Autodesk Inventor part; units mm, degrees
ref_plane "YZ Plane" through (0, 0, 0) normal (1, 0, 0) x (0, 1, 0)
ref_plane "XZ Plane" through (0, 0, 0) normal (0, 1, 0) x (-1, 0, 0)
ref_plane "XY Plane" through (0, 0, 0) normal (0, 0, 1) x (1, 0, 0)
sketch "Sketch1" plane through (0, 0, 0) normal (0, 1, 0) x (-1, 0, 0)
  arc A0 (740.7704, 834.1348) -> (40.7704, 134.1348) centre (740.7704, 134.1348) ccw
  line L0 (740.7704, 134.1348) -> (40.7704, 134.1348)
  line L1 (740.7704, 134.1348) -> (740.7704, 834.1348)
  line L2 (909.7653, 0) -> (-273.1993, 0)
  dimension "d2" = 1400
extrude "Extrusion1" add sketch "Sketch1" along normal blind 150
sketch "Sketch2" plane through (0, 0, 0) normal (0, -1, 0) x (1, 0, 0)
  arc A0 (-40.7704, 134.1348) -> (-740.7704, 834.1348) centre (-740.7704, 134.1348) ccw
  line L0 (-740.7704, 134.1348) -> (-740.7704, 834.1348)
  line L1 (-40.7704, 134.1348) -> (-740.7704, 134.1348)
  arc A1 (59.2296, 134.1348) -> (-740.7704, 934.1348) centre (-740.7704, 134.1348) ccw
  arc A2 (-40.7704, 134.1348) -> (-740.7704, 834.1348) centre (-740.7704, 134.1348) ccw
  line L2 (-40.7704, 134.1348) -> (59.2296, 134.1348)
  line L3 (-740.7704, 834.1348) -> (-740.7704, 934.1348)
  point P0 (0, 0)
  dimension "d5" = 100
extrude "Extrusion2" add sketch "Sketch2" against normal blind 200 contours A0 L3 A1 L2
properties part number "McCrea_zakruta_walle"
Read the model definition and answer for the solid it produces. Units are mm, in the model's axes. A direction names the side the tool comes from. Coordinates: 2 decimals unless noted, no trailing zeros. Loops run counter-clockwise (first coordinate to the right, second up) from the corner with the lowest first, then second, coordinate; pieces in that order, holes last.
Q1. Each of these flat-tipped pins is pushed along its axis until it touches: pin 1 Ø2 at (x, z) = (-327, 292.5) entering from +Y; pin 2 Ø4 at (y, z) = (70, 373.5) entering from +X; pin 3 Ø5 at (x, z) = (-550, 433.5) entering from -Y; pin 4 Ø12 at (x, y) = (-257.5, 112) entering from +Z. Where does it stop, or does it pass through?
Q2. Consider probe 1 along Y at (x, z) = (-253, 496); probe 2 along X at (y, z) = (93.5, 435.5); probe 3 along Z at (x, y) = (-382, 133). Determine where each line is inside the solid, lowest interval first.
Q3. The part is cut by section B-B on x = -101. Write down the section's boundary in (y, z).
Q4. Which of the six approach directions +Z, -Z, +X, -X, +Y, -Y give full straight-line access (tool end or side, diameter ignored) to faces 1 (the face through (-168.899, 98.6, 693.566)), 2 (the face through (-464, 150, 411))?
Q5. The part is cut by section C-C on y = 15. Write down the section's boundary in (x, z), and give its area (3 significant figures).
Q6. The part is cut by section A-A on z = 258. Write down the section's boundary in (x, y).
Results below:
1. pin 1: stops at y = 150
1. pin 2: stops at x = 23.2
1. pin 3: stops at y = 0
1. pin 4: stops at z = 776.17
2. probe 1: y = 0 to 150
2. probe 2: x = -740.77 to 0.3
2. probe 3: z = 134.13 to 849.18
3. outline: (0, 134.13) - (150, 134.13) - (150, 418.2) - (200, 418.2) - (200, 614.44) - (0, 614.44) - close
4. face 1: +Z, +X, +Y, -Y
4. face 2: -Z, -X, +Y
5. outline: (-740.77, 134.13) - (59.23, 134.13) arc R800 ccw to (-740.77, 934.13) - close
5. area: 503,000 mm2
6. outline: (-740.77, 0) - (49.58, 0) - (49.58, 200) - (-51.82, 200) - (-51.82, 150) - (-740.77, 150) - close
